Here's how the part is built. I have some questions about the finished solid (model axes, mm). Face numbers are marked on the shaded views. A direction names the side the tool comes from. Give positions to 0.01 mm unless a question says otherwise; leave off trailing zeros. Order: outer loops, then holes, each group sorted by start corner. A loop starts at its lowest first (then second) coordinate and runs counter-clockwise, first axis right, second up. Notation, with made-up numbers: (59.25, -34) -> (81.25, -34) arc R11 cw to (81.25, -21) -> close; hole circle Ø4 at (30, 61.25). An arc over 180 degrees is marked (long way). Write each question's results on one line, items separated by ' | '. Start each with the question number.
Q1. Thinking about a two-plate mould opening in Z: for the marked faces 1, 2, 3 and 4, which applies, pulls with the +Z half, pulls with the -Z half, needs draft (parallel to the pull), parting line crosses it, or undercut?
Q2. Imagine slicing it at B-B, the plane z = -0.75. Please give me the cut outline in (x, y).
Q3. Imagine slicing it at C-C, the plane x = 2.75. State how many separate pieces and enclosed holes the cut face has, then the cut area to 3 significant figures.
Q4. Imagine slicing it at A-A, the plane y = -3. Please give me the cut outline in (x, z), then the cut area to 3 significant figures.
Q5. Imagine slicing it at D-D, the plane z = 3. Please give me the cut outline in (x, y).
Q6. I need wall thicknesses on line 1 along Z through (x, y) = (4, -3); line 2 along Y through (x, z) = (3.25, 1.25); line 3 along Z through (x, y) = (2.5, 9.5). Which ranges of each line are inside material? Lowest first, please. Write a range as [from, to].
Q7. For the marked faces 5 and 6, which set-ups out of +Z, -Z, +X, -X, +Y, -Y let a thin tool reach every point of the face, with its end or its side?
Q8. I'm going to push flat-ended pins straight in: pin 1 (3.5 mm diameter, centred on y = -3, z = 0, fed in from -X); pin 2 (6 mm diameter, centred on x = 2.5, y = -24, fed in from +Z); pin 3 (1 mm diameter, centred on x = 5.5, z = 0.5, fed in from +Y) (3 decimals); pin 4 (5 mm diameter, centred on x = 9, z = 1, fed in from +Y). Where does each tip first touch, or does it pass through?
```python
from build123d import *

# Parameters (mm, degrees)
CYLINDER033_R             = 2
CYLINDER033_DEPTH         = 10
CYLINDER031_R             = 2
CYLINDER031_DEPTH         = 10
CYLINDER032_R             = 1
CYLINDER032_DEPTH         = 10
BOX031_W                  = 3
BOX031_H                  = 20
BOX031_DEPTH              = 10
BOX032_W                  = 1
BOX032_H                  = 15
BOX032_DEPTH              = 10
BOX032_PLACEMENT_ANGLE    = 30
BOX033_W                  = 3.3
BOX033_H                  = 8
BOX033_DEPTH              = 10
BOX033_PLACEMENT_ANGLE    = 30
CYLINDER029_R             = 2
CYLINDER029_DEPTH         = 10
CYLINDER030_R             = 4
CYLINDER030_DEPTH         = 10
FUSION024_PLACEMENT_ANGLE = 180
CYLINDER027_R             = 2
CYLINDER027_DEPTH         = 10
CYLINDER028_R             = 1
CYLINDER028_DEPTH         = 10
BOX028_W                  = 3
BOX028_H                  = 22
BOX028_DEPTH              = 10
BOX029_W                  = 1
BOX029_H                  = 15
BOX029_DEPTH              = 10
BOX029_PLACEMENT_ANGLE    = 30
BOX030_W                  = 3.3
BOX030_H                  = 8
BOX030_DEPTH              = 10
BOX030_PLACEMENT_ANGLE    = 30
CYLINDER025_R             = 2
CYLINDER025_DEPTH         = 10
CYLINDER026_R             = 4
CYLINDER026_DEPTH         = 10
FUSION026_PITCH_ANGLE     = 90


with BuildPart() as zylinder024:
    # Cylinder033 → Cylinder033 (new body)
    with BuildSketch(Plane(origin=(2, -7, 0), x_dir=(1, 0, 0), z_dir=(0, 0, 1))):
        Circle(CYLINDER033_R)
    extrude(amount=CYLINDER033_DEPTH)


with BuildPart() as zylinder022:
    # Cylinder031 → Cylinder031 (new body)
    with BuildSketch(Plane(origin=(2, -15, 0), x_dir=(1, 0, 0), z_dir=(0, 0, 1))):
        Circle(CYLINDER031_R)
    extrude(amount=CYLINDER031_DEPTH)


with BuildPart() as zylinder023:
    # Cylinder032 → Cylinder032 (new body)
    with BuildSketch(Plane(origin=(-2.73, -12.5, 0), x_dir=(1, 0, 0), z_dir=(0, 0, 1))):
        Circle(CYLINDER032_R)
    extrude(amount=CYLINDER032_DEPTH)


with BuildPart() as obj1:
    # Box031 → Box031 (new body)
    with BuildSketch(Plane(origin=(2, -28, 0), x_dir=(1, 0, 0), z_dir=(0, 0, 1))):
        with Locations((1.5, 10)):
            Rectangle(BOX031_W, BOX031_H)
    extrude(amount=BOX031_DEPTH)


with BuildPart() as obj2:
    # Box032 → Box032 (new body)
    with BuildSketch(Plane.XY):
        with Locations((0.5, 7.5)):
            Rectangle(BOX032_W, BOX032_H)
    extrude(amount=BOX032_DEPTH)


with BuildPart() as obj2_1:
    # Box032 placement: moved
    add(obj2.part.moved(Location((3.9, -26, 0))).rotate(Axis((3.9, -26, 0), (0, 0, 1)), BOX032_PLACEMENT_ANGLE))


with BuildPart() as obj3:
    # Box033 → Box033 (new body)
    with BuildSketch(Plane.XY):
        with Locations((1.65, 4)):
            Rectangle(BOX033_W, BOX033_H)
    extrude(amount=BOX033_DEPTH)


with BuildPart() as obj3_1:
    # Box033 placement: moved
    add(obj3.part.moved(Location((2, -21.5, 0))).rotate(Axis((2, -21.5, 0), (0, 0, 1)), BOX033_PLACEMENT_ANGLE))


with BuildPart() as zylinder020:
    # Cylinder029 → Cylinder029 (new body)
    with BuildSketch(Plane.XY):
        Circle(CYLINDER029_R)
    extrude(amount=CYLINDER029_DEPTH)


with BuildPart() as fusion024:
    # Cylinder030 → Cylinder030 (new body)
    with BuildSketch(Plane.XY):
        Circle(CYLINDER030_R)
    extrude(amount=CYLINDER030_DEPTH)

    # Cut010: cut Zylinder020
    add(zylinder020.part, mode=Mode.SUBTRACT)


with BuildPart() as fusion024_1:
    # Cut010 placement: moved
    add(fusion024.part.moved(Location((0, -11, 0))))

    # Fusion024: union Zylinder022, Zylinder023, obj1, obj2, obj3
    add(zylinder022.part)
    add(zylinder023.part)
    add(obj1.part)
    add(obj2_1.part)
    add(obj3_1.part)


with BuildPart() as fusion024_2:
    # Fusion024 placement: moved
    add(fusion024_1.part.moved(Location((0, -14, 10))).rotate(Axis((0, -14, 10), (1, 0, 0)), FUSION024_PLACEMENT_ANGLE))


with BuildPart() as zylinder018:
    # Cylinder027 → Cylinder027 (new body)
    with BuildSketch(Plane(origin=(2, -15, 0), x_dir=(1, 0, 0), z_dir=(0, 0, 1))):
        Circle(CYLINDER027_R)
    extrude(amount=CYLINDER027_DEPTH)


with BuildPart() as zylinder019:
    # Cylinder028 → Cylinder028 (new body)
    with BuildSketch(Plane(origin=(-2.73, -12.5, 0), x_dir=(1, 0, 0), z_dir=(0, 0, 1))):
        Circle(CYLINDER028_R)
    extrude(amount=CYLINDER028_DEPTH)


with BuildPart() as obj4:
    # Box028 → Box028 (new body)
    with BuildSketch(Plane(origin=(2, -28, 0), x_dir=(1, 0, 0), z_dir=(0, 0, 1))):
        with Locations((1.5, 11)):
            Rectangle(BOX028_W, BOX028_H)
    extrude(amount=BOX028_DEPTH)


with BuildPart() as obj5:
    # Box029 → Box029 (new body)
    with BuildSketch(Plane.XY):
        with Locations((0.5, 7.5)):
            Rectangle(BOX029_W, BOX029_H)
    extrude(amount=BOX029_DEPTH)


with BuildPart() as obj5_1:
    # Box029 placement: moved
    add(obj5.part.moved(Location((3.9, -26, 0))).rotate(Axis((3.9, -26, 0), (0, 0, 1)), BOX029_PLACEMENT_ANGLE))


with BuildPart() as obj6:
    # Box030 → Box030 (new body)
    with BuildSketch(Plane.XY):
        with Locations((1.65, 4)):
            Rectangle(BOX030_W, BOX030_H)
    extrude(amount=BOX030_DEPTH)


with BuildPart() as obj6_1:
    # Box030 placement: moved
    add(obj6.part.moved(Location((2, -21.5, 0))).rotate(Axis((2, -21.5, 0), (0, 0, 1)), BOX030_PLACEMENT_ANGLE))


with BuildPart() as zylinder016:
    # Cylinder025 → Cylinder025 (new body)
    with BuildSketch(Plane.XY):
        Circle(CYLINDER025_R)
    extrude(amount=CYLINDER025_DEPTH)


with BuildPart() as fusion026:
    # Cylinder026 → Cylinder026 (new body)
    with BuildSketch(Plane.XY):
        Circle(CYLINDER026_R)
    extrude(amount=CYLINDER026_DEPTH)

    # Cut009: cut Zylinder016
    add(zylinder016.part, mode=Mode.SUBTRACT)


with BuildPart() as fusion026_1:
    # Cut009 placement: moved
    add(fusion026.part.moved(Location((0, -11, 0))))

    # Fusion023: union Zylinder018, Zylinder019, obj4, obj5, obj6
    add(zylinder018.part)
    add(zylinder019.part)
    add(obj4.part)
    add(obj5_1.part)
    add(obj6_1.part)

    # Fusion025: union Fusion024
    add(fusion024_2.part)

    # Fusion026: union Zylinder024
    add(zylinder024.part)


with BuildPart() as fusion026_2:
    # Fusion026 pitch: moved
    add(fusion026_1.part.rotate(Axis((0, 0, 0), (0, 1, 0)), FUSION026_PITCH_ANGLE))


with BuildPart() as fusion026_3:
    # Fusion026 placement: moved
    add(fusion026_2.part)


solid = fusion026_3.part
```
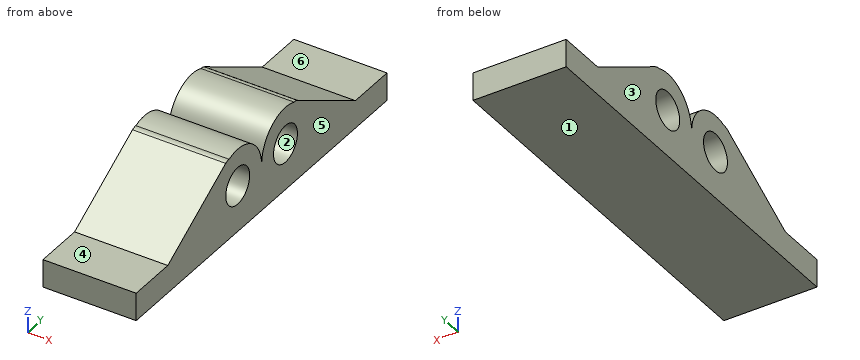
Geometry check:
1) face 1: pulls with the -Z half | face 2: undercut | face 3: needs draft | face 4: pulls with the +Z half
2) outline: (0, -20.54) -> (10, -20.54) -> (10, -12.85) -> (0, -12.85) -> close; (0, -9.15) -> (10, -9.15) -> (10, -4.85) -> (0, -4.85) -> close; (0, -1.15) -> (10, -1.15) -> (10, 6.54) -> (0, 6.54) -> close
3) separate pieces: 1 | enclosed holes: 2 | area: 220 mm²
4) outline: (0, -5) -> (10, -5) -> (10, -2) -> (0, -2) -> close; (0, 2) -> (10, 2) -> (10, 4) -> (0, 4) -> close | area: 50.0 mm²
5) outline: (0, -14.05) -> (10, -14.05) -> (10, -8.35) -> (0, -8.35) -> close; (0, -5.65) -> (10, -5.65) -> (10, 0.05) -> (0, 0.05) -> close
6) line 1: [-5, -2], [2, 4] | line 2: [-17.08, -12.56], [-9.44, -7.2], [-6.8, -4.56], [-1.44, 3.08] | line 3: [-5, -2]
7) face 5: +Z, -Z, +X, +Y, -Y | face 6: +Z, +X, -X, +Y
8) pin 1: through | pin 2: z = -1.01 | pin 3: y = 5.245 | pin 4: y = 7.84
